Source: CAD feature listing. Evaluate the final solid. Frame: model axes, mm. A direction names the side the tool comes from. Round coordinates to 2 decimals unless told otherwise and drop trailing zeros. Loops run counter-clockwise (first coordinate to the right, second up) from the corner with the lowest first, then second, coordinate; pieces in that order, holes last. Notation, with made-up numbers: (0, 86) - (4, 86) arc R20 ccw to (4, 119) - close; hole circle Ø8 at (88, 41.5). An arc over 180 degrees is marked (long way). One line per question, with ' | ' between items.
from build123d import *

# Parameters (mm, degrees)
MODEL_W             = 185
MODEL_H             = 150
MODEL_R             = 3.05
MODEL_W_2           = 20
MODEL_H_2           = 8
MODEL_W_3           = 8
MODEL_H_3           = 20
BOSS_EXTRUDE1_DEPTH = 8


with BuildPart() as part:
    # Model → Boss-Extrude1 (new body)
    with BuildSketch(Plane.XY):
        with Locations((77.5, 60)):
            Rectangle(MODEL_W, MODEL_H)
        with Locations((77.5, -4)):
            Circle(MODEL_R, mode=Mode.SUBTRACT)
        with Locations((-4, 110)):
            Circle(MODEL_R, mode=Mode.SUBTRACT)
        with Locations((-4, 25)):
            Circle(MODEL_R, mode=Mode.SUBTRACT)
        with Locations((25, -4)):
            Circle(MODEL_R, mode=Mode.SUBTRACT)
        with Locations((130, -4)):
            Circle(MODEL_R, mode=Mode.SUBTRACT)
        with Locations((51.25, -4)):
            Rectangle(MODEL_W_2, MODEL_H_2, mode=Mode.SUBTRACT)
        with Locations((103.75, -4)):
            Rectangle(MODEL_W_2, MODEL_H_2, mode=Mode.SUBTRACT)
        with BuildLine():
            Line((40, 45), (40, 70))
            ThreePointArc((40, 70), (80, 110), (120, 70))
            Line((120, 70), (120, 45))
            ThreePointArc((120, 45), (80, 5), (40, 45))
        make_face(mode=Mode.SUBTRACT)
        with Locations((-4, 88.75)):
            Rectangle(MODEL_W_3, MODEL_H_3, mode=Mode.SUBTRACT)
        with Locations((-4, 46.25)):
            Rectangle(MODEL_W_3, MODEL_H_3, mode=Mode.SUBTRACT)
    extrude(amount=BOSS_EXTRUDE1_DEPTH)


solid = part.part
1. Section query A-A, the plane x = 130. Return loops of the section in (y, z), plus the area to 3 significant figures.
Worked out:
outline: (-15, 0) - (-7.05, 0) - (-7.05, 8) - (-15, 8) - close; (-0.95, 0) - (135, 0) - (135, 8) - (-0.95, 8) - close | area: 1,150 mm2
2. Access query for faces 5 (the flat face through (35, 61, 8)), 6 (the flat face through (-4, 36.25, 4)). Directions: +Z, -Z, +X, -X, +Y, -Y. A direction counts if a zero-diameter tool reaches every point of the face in a straight line with its end or side. Return the directions, or none.
Worked out:
face 5: +Z, +X, -X, +Y, -Y | face 6: +Z, -Z
3. Contact query for a flat-ended pin moving along its axis: P1, Ø5, axis at x = -4, y = 110, coming from the -Z side. Output: stop coordinate, or through.
Worked out:
P1: passes through
4. Section query D-D, the plane x = 77.5. Return loops of the section in (y, z), plus the area to 3 significant figures.
Worked out:
outline: (-15, 0) - (-7.05, 0) - (-7.05, 8) - (-15, 8) - close; (-0.95, 0) - (5.08, 0) - (5.08, 8) - (-0.95, 8) - close; (109.92, 0) - (135, 0) - (135, 8) - (109.92, 8) - close | area: 312 mm2
5. Mould query, pull axis X, two halves, no side actions, for faces 1 (the flat face through (76, -15, 4)), 2 (the cylindrical face through (27.817, -5.168, 3.944)), 3 (the flat face through (-15, 59, 4)), 4 (the flat face through (51, 0, 4)). Classes: released by +X, released by -X, zero draft, split by the parting line, or undercut.
Worked out:
face 1: zero draft | face 2: undercut | face 3: released by -X | face 4: undercut
6. Section query B-B, the plane z = 1.5. Give the number of separate pieces and of enclosed holes in the cut face, plus the area to 3 significant figures.
Worked out:
separate pieces: 1 | enclosed holes: 10 | area: 19,900 mm2
7. Section query C-C, the plane y = 60.5. Return loops of the section in (x, z), plus the area to 3 significant figures.
Worked out:
outline: (-15, 0) - (40, 0) - (40, 8) - (-15, 8) - close; (120, 0) - (170, 0) - (170, 8) - (120, 8) - close | area: 840 mm2
8. Material intervals for probe 1 along Y at (x, z) = (-4, 4); probe 2 along X at (y, z) = (68, 4); probe 3 along Y at (x, z) = (81, 6.5), sorted ascending.
Worked out:
probe 1: y = -15 to 21.95, 28.05 to 36.25, 56.25 to 78.75, 98.75 to 106.95, 113.05 to 135 | probe 2: x = -15 to 40, 120 to 170 | probe 3: y = -15 to 5.01, 109.99 to 135
